Drawing for the job (mm, zero at the part's lowest x, y, z). A direction names the side the tool comes from. Round coordinates to 2 decimals unless told otherwise and drop trailing zeros. Order: outer loops, then holes, each group sorted by start corner. A loop starts at its lowest first (then second) coordinate and runs counter-clockwise, first axis right, second up. Notation, with made-up numbers: M -11,60 L 48,60 A20 cw 48,64 Z; hole C 18,60 d2. An arc over 180 degrees is marked long. One line per item, written item: value. Start each with the question number.
Item 1: Band-saw the part on C-C, the plane y = 8. Write the cut outline in (x, z).
Item 2: Band-saw the part on A-A, the plane z = 10. Give the number of separate pieces and of enclosed holes in the cut face, then the cut area to 3 significant figures.
Item 3: Two-plate mould, pull along X, no slides. Class the marked faces 1, 2, 3 and 4: +X half, -X half, draft (parallel to the pull), parting line (faces both ways), or undercut.
Item 4: Band-saw the part on B-B, the plane x = 44. Write the cut outline in (y, z), then the cut area to 3 significant figures.
Item 5: Probe L1, parallel to X at y = 19, z = 44 (1 decimal); L2, parallel to Y at x = 71, z = 40; L3, parallel to X at y = 32, z = 9. List the from-to ranges inside material, lowest first.
Item 6: Pin check, flat tips, straight feed: pin 1 (4 mm diameter, centred on x = 3.5, z = 32.5, fed in from -Y); pin 2 (7.5 mm diameter, centred on x = 71.44, y = 19.05, fed in from +Z); pin 3 (1 mm diameter, centred on x = 26.5, z = 13.5, fed in from +Y). Stop position of each tip, or through.
Item 7: Tool access for the marked faces 5, 6 and 7: list every direction of +Z, -Z, +X, -X, +Y, -Y with a clear straight run to the whole face (end or side of a thin tool).
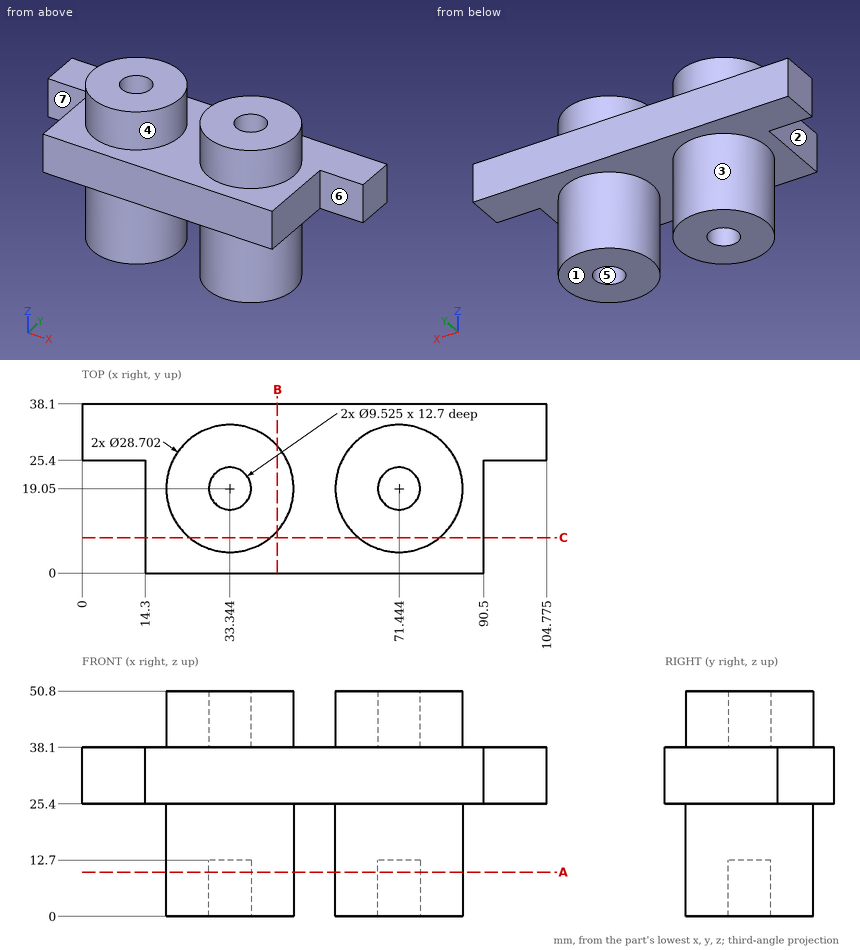
Output:
1. outline: M 14.3,25.4 L 24.19,25.4 L 24.19,0 L 42.5,0 L 42.5,25.4 L 62.29,25.4 L 62.29,0 L 80.6,0 L 80.6,25.4 L 90.5,25.4 L 90.5,38.1 L 80.6,38.1 L 80.6,50.8 L 62.29,50.8 L 62.29,38.1 L 42.5,38.1 L 42.5,50.8 L 24.19,50.8 L 24.19,38.1 L 14.3,38.1 Z
2. separate pieces: 2
2. enclosed holes: 2
2. area: 1,150 mm²
3. face 1: draft
3. face 2: -X half
3. face 3: undercut
3. face 4: undercut
4. outline: M 0,25.4 L 9.44,25.4 L 9.44,0 L 28.66,0 L 28.66,25.4 L 38.1,25.4 L 38.1,38.1 L 28.66,38.1 L 28.66,50.8 L 9.44,50.8 L 9.44,38.1 L 0,38.1 Z
4. area: 1,220 mm²
5. L1: x = 19 to 28.6, 38.1 to 47.7, 57.1 to 66.7, 76.2 to 85.8
5. L2: y = 4.71 to 14.31, 23.79 to 33.39
5. L3: x = 27.16 to 39.53, 65.26 to 77.63
6. pin 1: stops at y = 25.4
6. pin 2: stops at z = 38.1
6. pin 3: stops at y = 31.92
7. face 5: -Z
7. face 6: +Z, -Z, +X, -Y
7. face 7: +Z, -Z, -X, -Y
